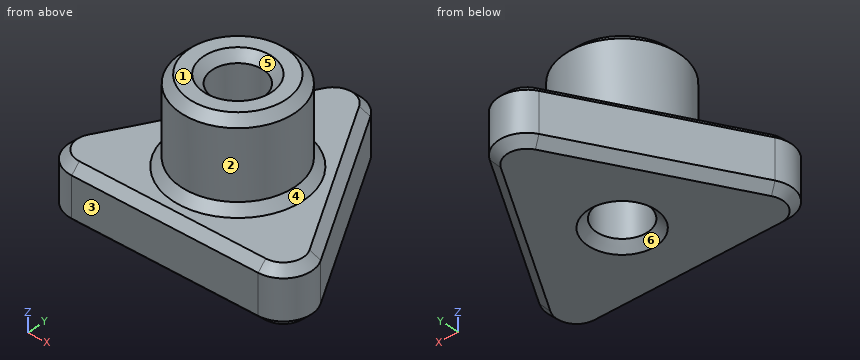
```python
from build123d import *

# Parameters (mm, degrees)
F1_DEPTH = 5.08
F2_R     = 5.08
F3_DEPTH = 12.7
F4_D     = 4.572
F5_R     = 2.54
F6_SIZE  = 0.762


with BuildPart() as f1:
    # F0 (on Top) → F1 (new body)
    with BuildSketch(Plane.XY):
        Polygon((12.7, -7.3323484187), (0, 14.6646968374), (-12.7, -7.3323484187), align=None)
    extrude(amount=F1_DEPTH)

    # F2 (on Top) → F3 (join)
    with BuildSketch(Plane.XY):
        Circle(F2_R)
    extrude(amount=F3_DEPTH)

    # F4 (through all)
    with Locations(Plane(origin=(0, 0, 0), x_dir=(1, 0, 0), z_dir=(0, 0, -1))):
        with Locations((0, 0)):
            Hole(F4_D / 2)

    # F5
    f5_edges = [f1.edges().sort_by_distance(p)[0] for p in [
        (-12.7, -7.332348, 2.54),
        (12.7, -7.332348, 2.54),
        (0, 14.664697, 2.54),
    ]]
    fillet(f5_edges, radius=F5_R)

    # F6
    f6_edges = [f1.edges().sort_by_distance(p)[0] for p in [
        (6.35, 3.666174, 0),
        (10.500295, -6.062348, 0),
        (0, 12.124697, 0),
        (0, -7.332348, 0),
        (-6.35, 3.666174, 0),
        (-10.500295, -6.062348, 0),
        (-2.286, 0, 0),
        (-5.08, 0, 12.7),
        (-2.286, 0, 12.7),
        (6.35, 3.666174, 5.08),
        (10.500295, -6.062348, 5.08),
        (0, 12.124697, 5.08),
        (0, -7.332348, 5.08),
        (-6.35, 3.666174, 5.08),
        (-10.500295, -6.062348, 5.08),
        (-5.08, 0, 5.08),
    ]]
    chamfer(f6_edges, length=F6_SIZE)


solid = f1.part
```
Verification items for the finished model (mm, model axes). Face numbers are marked on the shaded views. A direction names the side the tool comes from. Give positions to 0.01 mm unless a question says otherwise; leave off trailing zeros. Loops run counter-clockwise (first coordinate to the right, second up) from the corner with the lowest first, then second, coordinate; pieces in that order, holes last.
1. Section check B-B, the plane z = 1.75. Enter the section's corners in (x, y).
2. Section check C-C, the plane y = 0. Enter the section's corners in (x, z), then the cut area to 3 significant figures.
3. Mould release check, pull along X, two halves, no side actions. Record for the marked faces 3, 4, 5 and 6: released by +X, released by -X, zero draft, split by the parting line, or undercut.
4. Thickness scan on line 1 (X direction, y = 0, z = 9.25); line 2 (Z direction, x = -3.5, y = 5.5). Record the ranges inside material, lowest first.
5. Section check A-A, the plane x = 0. Enter the section's corners in (y, z).
6. Section check D-D, the plane y = 7.25. Enter the section's corners in (x, z).
7. Set-up check for the marked faces 1 and 2: record each of +Z, -Z, +X, -X, +Y, -Y from which the full face is reachable in a straight line by a thin tool's end or side.
8. Go/stop test with flat-tipped pins: pin 1 Ø3 at (y, z) = (7, 10) entering from -X; pin 2 Ø5.5 at (x, y) = (3, 3.5) entering from +Z; pin 3 Ø4 at (y, z) = (1, 7.5) entering from -X; pin 4 Ø5 at (x, y) = (5, 5.5) entering from +Z. Record where each tip stops, or that it passes through.
Geometry says:
1. outline: (-10.5, -3.52) arc R2.54 ccw to (-8.3, -7.33) - (8.3, -7.33) arc R2.54 ccw to (10.5, -3.52) - (2.2, 10.85) arc R2.54 ccw to (-2.2, 10.85) - close; hole circle Ø4.57 at (0, 0)
2. outline: (-8.47, 0.76) - (-7.59, 0) - (-3.05, 0) - (-2.29, 0.76) - (-2.29, 11.94) - (-3.05, 12.7) - (-4.32, 12.7) - (-5.08, 11.94) - (-5.08, 5.84) - (-5.84, 5.08) - (-7.59, 5.08) - (-8.47, 4.32) - close; (2.29, 0.76) - (3.05, 0) - (7.59, 0) - (8.47, 0.76) - (8.47, 4.32) - (7.59, 5.08) - (5.84, 5.08) - (5.08, 5.84) - (5.08, 11.94) - (4.32, 12.7) - (3.05, 12.7) - (2.29, 11.94) - close
2. area: 103 mm2
3. face 3: zero draft
3. face 4: split by the parting line
3. face 5: undercut
3. face 6: undercut
4. line 1: x = -5.08 to -2.29, 2.29 to 5.08
4. line 2: z = 0 to 5.08
5. outline: (-7.33, 0.76) - (-6.57, 0) - (-3.05, 0) - (-2.29, 0.76) - (-2.29, 11.94) - (-3.05, 12.7) - (-4.32, 12.7) - (-5.08, 11.94) - (-5.08, 5.84) - (-5.84, 5.08) - (-6.57, 5.08) - (-7.33, 4.32) - close; (2.29, 0.76) - (3.05, 0) - (11.36, 0) - (12.12, 0.76) - (12.12, 4.32) - (11.36, 5.08) - (5.84, 5.08) - (5.08, 5.84) - (5.08, 11.94) - (4.32, 12.7) - (3.05, 12.7) - (2.29, 11.94) - close
6. outline: (-4.28, 0.76) - (-3.4, 0) - (3.4, 0) - (4.28, 0.76) - (4.28, 4.32) - (3.4, 5.08) - (-3.4, 5.08) - (-4.28, 4.32) - close
7. face 1: +Z, +X, -X, +Y, -Y
7. face 2: +Z
8. pin 1: passes through
8. pin 2: stops at z = 12.7
8. pin 3: stops at x = -5.35
8. pin 4: stops at z = 12.08
